Study the drawing (mm; zero at the part's minimum x, y, z) and answer. A direction names the side the tool comes from. Coordinates: 2 decimals unless noted, no trailing zeros. Write each loop counter-clockwise with the first axis right and the second up, starting at its lowest first coordinate (ties: lowest second). Pieces come first, ordered by that corner, then holes. Notation, with made-up numbers: (-9.5, 54) -> (19.5, 54) arc R22 ccw to (19.5, 69) -> close; hole circle Ø2 at (-12.5, 18). An arc over 180 degrees is marked (long way). Write each question's results on one line, items separated by ' | '. Start each with the question number.
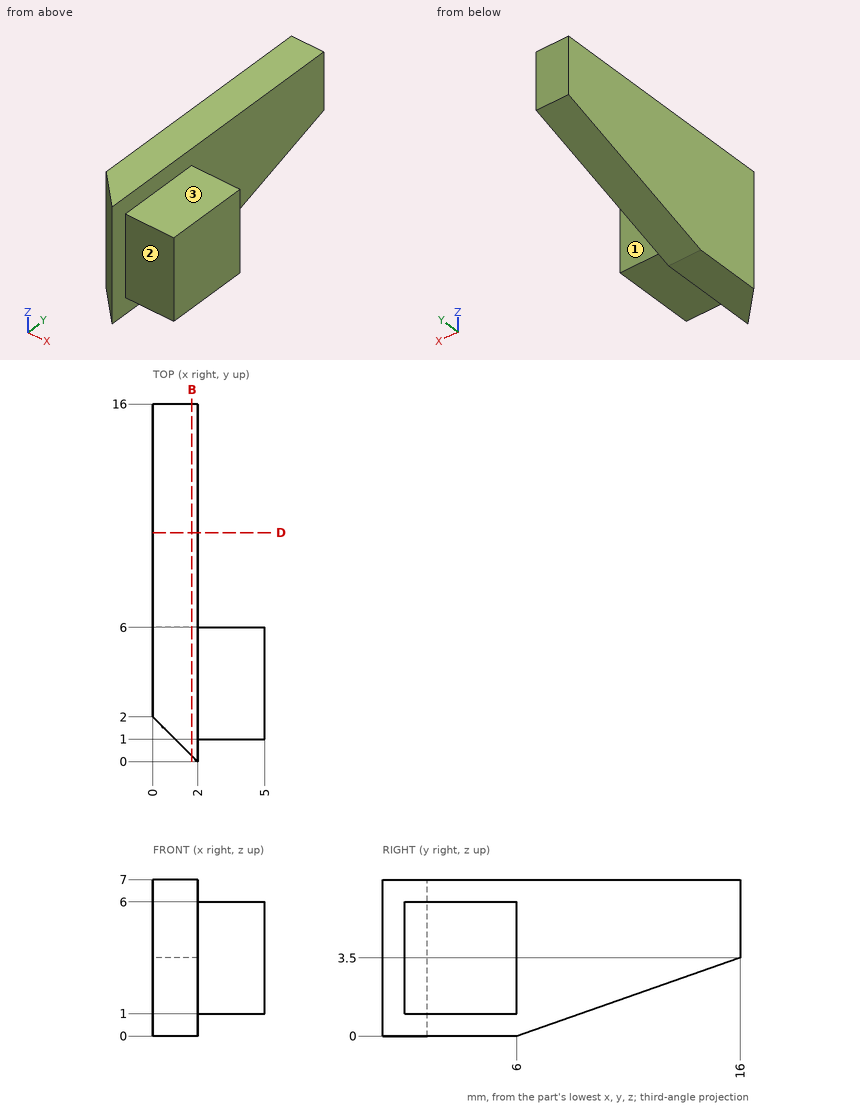
1. Given pin 1 Ø1.5 at (x, z) = (3, 3) entering from +Y; pin 2 Ø1.5 at (y, z) = (12, 2) entering from -X; pin 3 Ø2.5 at (x, z) = (3.5, 2.5) entering from -Y; pin 4 Ø1.5 at (x, y) = (3, 2.5) entering from -Z, each flat-ended and moving along its own axis, determine where each tip first touches the part or whether it passes through.
2. Find section B-B on x = 1.75. Give the vertices of the cut face in (y, z), and give its area (4 significant figures).
3. Find section D-D on y = 10.25. Give the vertices of the cut face in (x, z).
4. For the marked faces 1, 2 and 3, determine the directions among +Z, -Z, +X, -X, +Y, -Y from which every point of the face is accessible in a straight line to the end or side of a thin tool.
5. Find the intervals of material crossed by L1, parallel to X at y = 8.5, z = 6.25; L2, parallel to Y at x = 2.3, z = 5.5, in increasing order.
Ans:
1) pin 1: stops at y = 6 | pin 2: stops at x = 0 | pin 3: stops at y = 1 | pin 4: stops at z = 1
2) outline: (0.25, 0) -> (6, 0) -> (16, 3.5) -> (16, 7) -> (0.25, 7) -> close | area: 92.75 mm²
3) outline: (0, 1.49) -> (2, 1.49) -> (2, 7) -> (0, 7) -> close
4) face 1: +Z, -Z, +X, +Y | face 2: +Z, -Z, +X, -Y | face 3: +Z, +X, +Y, -Y
5) L1: x = 0 to 2 | L2: y = 1 to 6
